Work out the finished part from the listing and answer in its coordinate system (mm). A direction names the side the tool comes from. Round coordinates to 2 decimals unless told otherwise and drop trailing zeros. Loops run counter-clockwise (first coordinate to the right, second up) from the corner with the lowest first, then second, coordinate; pieces in that order, holes last.
Autodesk Inventor part; units mm, degrees
ref_plane "YZ Plane" through (0, 0, 0) normal (1, 0, 0) x (0, 1, 0)
ref_plane "XZ Plane" through (0, 0, 0) normal (0, 1, 0) x (-1, 0, 0)
ref_plane "XY Plane" through (0, 0, 0) normal (0, 0, 1) x (1, 0, 0)
sketch "Sketch1" plane through (0, 0, 0) normal (0, 0, 1) x (1, 0, 0)
  line L0 (-31, -31) -> (31, -31)
  line L1 (31, -31) -> (31, 31)
  line L2 (31, 31) -> (-31, 31)
  line L3 (-31, 31) -> (-31, -31)
  line L4 (-31, -31) -> (31, 31) construction
  line L5 (31, -31) -> (-31, 31) construction
  line L6 (-33, 33) -> (33, 33)
  line L7 (33, 33) -> (33, -33)
  line L8 (33, -33) -> (-33, -33)
  line L9 (-33, -33) -> (-33, 33)
  point P0 (0, 0)
  dimension "d0" = 62
  dimension "d1" = 62
  dimension "d2" = 2
extrude "Extrusion1" add sketch "Sketch1" along normal blind 2 contours L3 L2 L1 L0 | L6 L7 L8 L9
extrude "Extrusion2" add sketch "Sketch1" against normal blind 12
sketch "Sketch2" plane through (-33, 33, 2) normal (0, 1, 0) x (1, 0, 0)
  line L0 (13, 3) -> (53, 3)
  line L1 (53, 3) -> (53, 0)
  line L2 (53, 0) -> (13, 0)
  line L3 (13, 0) -> (13, 3)
  line L4 (0, 14) -> (0, 0)
  line L5 (0, 14) -> (66, 14)
  point P0 (33, 2)
  dimension "d7" = 40
  dimension "d8" = 3
  dimension "d9" = 13
  dimension "d10" = 11
extrude "Extrusion3" add sketch "Sketch2" along normal blind 12
sketch "Sketch3" plane through (20, 33, -1) normal (0, 0, -1) x (-1, 0, 0)
  line L0 (40, 12) -> (0, 12)
  line L1 (40, 0) -> (40, 12)
  line L2 (0, 12) -> (40, 12)
  line L3 (40, 12) -> (40, 9)
  line L4 (40, 9) -> (0, 9)
  line L5 (0, 9) -> (0, 12)
  point P0 (20, -33)
  dimension "d13" = 3
extrude "Extrusion4" add sketch "Sketch3" along normal blind 80
sketch "Sketch4" plane through (-20, 42, -1) normal (0, -1, 0) x (1, 0, 0)
  line L0 (30.5, -63) -> (9.5, -63)
  line L1 (9.5, -63) -> (9.5, -22)
  line L2 (9.5, -22) -> (30.5, -22)
  line L3 (30.5, -22) -> (30.5, -63)
  line L4 (40, 3) -> (40, -80)
  line L5 (0, 3) -> (40, 3)
  point P0 (20, 1)
  dimension "d16" = 21
  dimension "d17" = 41
  dimension "d18" = 9.5
  dimension "d19" = 25
extrude "Extrusion5" cut sketch "Sketch4" against normal blind 80
sketch "Sketch5" plane through (-20, 42, -1) normal (0, -1, 0) x (1, 0, 0)
  line L0 (30.5, -63) -> (9.5, -63)
  line L1 (30.5, -63) -> (9.5, -63)
  line L2 (9.5, -63) -> (9.5, -69.81)
  line L3 (9.5, -69.81) -> (30.5, -69.81)
  line L4 (30.5, -69.81) -> (30.5, -63)
  circle A0 centre (14.45, -67.61) radius 2.25
  line L5 (30.5, -22) -> (30.5, -63)
  line L6 (30.5, -22) -> (9.5, -22)
  line L7 (9.5, -22) -> (9.5, -15.19)
  line L8 (9.5, -15.19) -> (30.5, -15.19)
  line L9 (30.5, -15.19) -> (30.5, -22)
  circle A1 centre (25.55, -17.39) radius 2.25
  point P0 (20, 1)
  point P1 (14.9217, -69.81)
  point P2 (13.9783, -69.81)
  point P3 (25.0783, -15.19)
  point P4 (26.0217, -15.19)
  dimension "d22" = 6.81
  dimension "d23" = 4.5
  dimension "d24" = 4.61
  dimension "d25" = 4.95
  dimension "d26" = 6.81
  dimension "d27" = 4.5
  dimension "d28" = 4.95
  dimension "d29" = 4.61
extrude "Extrusion6" cut sketch "Sketch5" against normal blind 80 contours L3 A0 | A1 L8 picked at (13.7855, -67.0048) picked at (26.1347, -16.9649)
properties part number "pan_base_holder"
1. Determine the mould class of faces 6 (the face through (-3, -32, -12)), 7 (the face through (13, 45, -39)), 8 (the face through (0, 31, -6)) for opening direction Y: +Y half, -Y half, draft (parallel to the pull), parting line (faces both ways), or undercut.
Answer key:
face 6: draft
face 7: +Y half
face 8: undercut
2. Given pin 1 (2 mm diameter, centred on x = 17, z = -47.5, fed in from -Y); pin 2 (10 mm diameter, centred on x = -21, y = 22.5, fed in from -Z); pin 3 (6 mm diameter, centred on x = -10, y = 34.5, fed in from -Z), each flat-ended and moving along its own axis, determine where each tip first touches the part or whether it passes through.
Answer key:
pin 1: stops at y = 42
pin 2: stops at z = 0
pin 3: stops at z = -12
3. Consider probe 1 along Z at (x, y) = (5.55, 42.9); probe 2 along Z at (x, y) = (-5.55, 43.85); probe 3 along X at (y, z) = (43.3, -18.39). Determine where each line is inside the solid, lowest interval first.
Answer key:
probe 1: z = -81 to -64, -23 to -20.64, -16.19 to 2
probe 2: z = -81 to -70.81, -66.36 to -64, -23 to 2
probe 3: x = -20 to 3.3, 7.8 to 20
4. Find section D-D (x = 16). Write down the section's boundary in (y, z), then the cut area to 3 significant figures.
Answer key:
outline: (-33, -12) - (-31, -12) - (-31, 0) - (31, 0) - (31, -12) - (33, -12) - (33, -1) - (42, -1) - (42, -81) - (45, -81) - (45, 2) - (-33, 2) - close
area: 456 mm2
5. Find section C-C (y = -24). Write down the section's boundary in (x, z), then the cut area to 3 significant figures.
Answer key:
outline: (-33, -12) - (-31, -12) - (-31, 0) - (31, 0) - (31, -12) - (33, -12) - (33, 2) - (-33, 2) - close
area: 180 mm2
6. Find section A-A (z = -62). Write down the section's boundary in (x, y), then the cut area to 3 significant figures.
Answer key:
outline: (-20, 42) - (-10.5, 42) - (-10.5, 45) - (-20, 45) - close; (10.5, 42) - (20, 42) - (20, 45) - (10.5, 45) - close
area: 57.0 mm2
7. Which of the six approach directions +Z, -Z, +X, -X, +Y, -Y give full straight-line access (tool end or side, diameter ignored) to faces 1 (the face through (-10.5, 43, -44)), 2 (the face through (0, 0, 0)), 3 (the face through (0, 37, -1)), 4 (the face through (-20, 43, -36)), 5 (the face through (20, 43, -36))?
Answer key:
face 1: +Y, -Y
face 2: -Z
face 3: -Z, +X, -X
face 4: +Z, -Z, -X, +Y
face 5: +Z, -Z, +X, +Y
8. Find section B-B (x = 1.5). Write down the section's boundary in (y, z).
Answer key:
outline: (-33, -12) - (-31, -12) - (-31, 0) - (31, 0) - (31, -12) - (33, -12) - (33, -1) - (42, -1) - (42, -23) - (45, -23) - (45, 2) - (-33, 2) - close; (42, -81) - (45, -81) - (45, -64) - (42, -64) - close
